from build123d import *

# Parameters (mm, degrees)
CORPO_DEPTH                 = 20
REBAIXO_SHCS_M4_D           = 4.5
REBAIXO_SHCS_M4_DEPTH       = 30
REBAIXO_SHCS_M4_CBORE_D     = 8
REBAIXO_SHCS_M4_CBORE_DEPTH = 4
REBAIXO_SHCS_M4_TIP         = 1.351936393


with BuildPart() as part:
    # Sketch1 → Corpo (new body)
    with BuildSketch(Plane.XY):
        with BuildLine():
            Line((16.252058195, 8.088672021), (23.764502557, 12.488672021))
            ThreePointArc((23.764502557, 12.488672021), (26.263743802, 12.734356122), (28.074119126, 10.993922652))
            ThreePointArc((28.074119126, 10.993922652), (30.15, 0), (28.074119126, -10.993922652))
            ThreePointArc((28.074119126, -10.993922652), (26.263743802, -12.734356122), (23.764502557, -12.488672021))
            Line((23.764502557, -12.488672021), (16.252058195, -8.088672021))
            ThreePointArc((16.252058195, -8.088672021), (14.971668435, -6.585929552), (14.902386515, -4.612903226))
            ThreePointArc((14.902386515, -4.612903226), (15.6, 0), (14.902386515, 4.612903226))
            ThreePointArc((14.902386515, 4.612903226), (14.971668435, 6.585929552), (16.252058195, 8.088672021))
        make_face()
    extrude(amount=CORPO_DEPTH)

    # Rebaixo SHCS M4
    with Locations(Plane.XY.offset(20)):
        with Locations((21.1, 0)):
            CounterBoreHole(REBAIXO_SHCS_M4_D / 2, REBAIXO_SHCS_M4_CBORE_D / 2, REBAIXO_SHCS_M4_CBORE_DEPTH, depth=REBAIXO_SHCS_M4_DEPTH)
            with Locations((0, 0, -(REBAIXO_SHCS_M4_DEPTH + REBAIXO_SHCS_M4_TIP / 2))):  # 118° drill point
                Cone(0, REBAIXO_SHCS_M4_D / 2, REBAIXO_SHCS_M4_TIP, mode=Mode.SUBTRACT)


solid = part.part
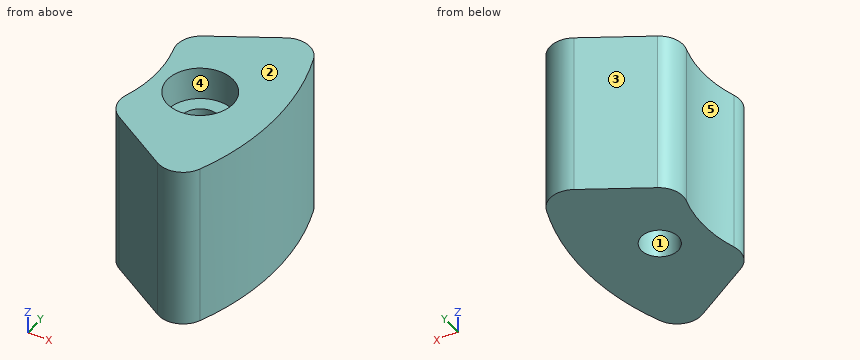
Build history of the part. All positions in model axes, mm. Face numbers are marked on the shaded views. A direction names the side the tool comes from. Coordinates: 2 decimals unless noted, no trailing zeros. Write each loop counter-clockwise with the first axis right and the second up, starting at its lowest first coordinate (ties: lowest second). Pieces come first, ordered by that corner, then holes. Notation, with made-up numbers: (-3, -30.75) -> (19, -30.75) arc R5 cw to (19, -21.75) -> close; hole circle Ø11 at (88.5, 54). An arc over 180 degrees is marked (long way). Use CSV: the item, a comma, the result in double quotes. Start each with the question number.
Q1. Cut at A-A, the plane y = 0. List the corners of the cut face in (x, z).
Q2. Cut at C-C, the plane x = 21.1. List the corners of the cut face in (y, z).
Q3. Cut at D-D, the plane y = -3. List the corners of the cut face in (x, z), then the cut area to 3 significant figures.
Q4. 3-axis set-ups, long thin cutter, end or side, ignore diameter. For the marked faces 4 and 5: which of +Z, -Z, +X, -X, +Y, -Y reach the whole face in a straight line?
Q5. Flat gauge pins, fed straight in: pin 1 Ø1.5 at (y, z) = (9, 17) entering from +X; pin 2 Ø6 at (x, z) = (18, 17.5) entering from -Y; pin 3 Ø9 at (x, y) = (21, 1.5) entering from +Z; pin 4 Ø3.5 at (x, y) = (21.1, 0) entering from +Z. Where does each tip first touch, or does it go through?
Q6. Drill centre lines: probe 1 along Y at (x, z) = (21.1, 4.5); probe 2 along Y at (x, z) = (21.1, 18.45); probe 3 along Z at (x, y) = (19, -2.5). Where is each one in solid material? Low to high.
Q7. Pull direction Y, two halves, no side cores. Call the marked faces 1, 2 and 3: released by +Y, released by -Y, zero draft, split by the parting line, or undercut.
Q8. Cut at B-B, the plane z = 4.75. List the corners of the cut face in (x, y).
Checked values:
1,outline,"(15.6, 0) -> (18.85, 0) -> (18.85, 16) -> (17.1, 16) -> (17.1, 20) -> (15.6, 20) -> close; (23.35, 0) -> (30.15, 0) -> (30.15, 20) -> (25.1, 20) -> (25.1, 16) -> (23.35, 16) -> close"
2,outline,"(-10.93, 0) -> (-2.25, 0) -> (-2.25, 16) -> (-4, 16) -> (-4, 20) -> (-10.93, 20) -> close; (2.25, 0) -> (10.93, 0) -> (10.93, 20) -> (4, 20) -> (4, 16) -> (2.25, 16) -> close"
3,outline,"(15.31, 0) -> (30, 0) -> (30, 20) -> (23.75, 20) -> (23.75, 16) -> (18.45, 16) -> (18.45, 20) -> (15.31, 20) -> close"
3,area,"273 mm²"
4,face 4,"+Z"
4,face 5,"+Z, -Z, -X"
5,pin 1,"stops at x = 29"
5,pin 2,"stops at y = -10.87"
5,pin 3,"stops at z = 20"
5,pin 4,"passes through"
6,probe 1,"y = -10.93 to -2.25, 2.25 to 10.93"
6,probe 2,"y = -10.93 to -4, 4 to 10.93"
6,probe 3,"z = 0 to 16"
7,face 1,"undercut"
7,face 2,"zero draft"
7,face 3,"released by +Y"
8,outline,"(14.9, -4.61) arc R3 ccw to (16.25, -8.09) -> (23.76, -12.49) arc R3 ccw to (28.07, -10.99) arc R30.15 ccw to (28.07, 10.99) arc R3 ccw to (23.76, 12.49) -> (16.25, 8.09) arc R3 ccw to (14.9, 4.61) arc R15.6 cw to start; hole circle Ø4.5 at (21.1, 0)"
